Check sheet for the drawn part. Datum: minimum x, y, z corner. Units: mm. A direction names the side the tool comes from. Coordinates: 2 decimals unless noted, no trailing zeros. Order: outer loops, then holes, each group sorted by start corner. A loop starts at its lowest first (then second) coordinate and runs counter-clockwise, first axis right, second up. Notation, with made-up numbers: (65, -12.75) -> (110, -12.75) arc R20 ccw to (110, 2.25) -> close; hole circle Ø11 at (-11.5, 5.5). An arc over 180 degrees is marked (long way). Write item = value, one per line. Start each with the question number.
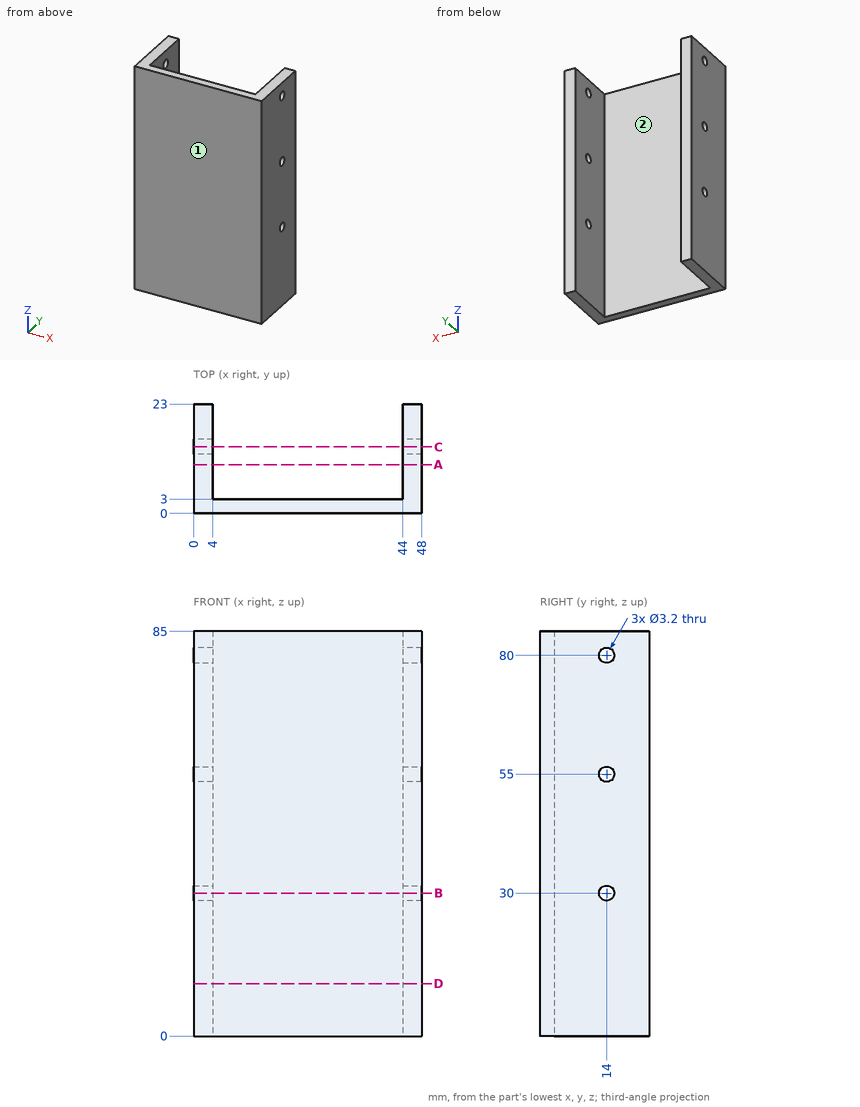
Item 1: Thickness scan on line 1 (Y direction, x = 2.7, z = 55); line 2 (X direction, y = 7, z = 33); line 3 (Y direction, x = 22.5, z = 27). Record the ranges inside material, lowest first.
Item 2: Section check C-C (y = 14). State how many separate pieces and enclosed holes the cut face has, then the cut area to 3 significant figures.
Item 3: Tool access check on the marked faces 1 and 2. Record the directions out of +Z, -Z, +X, -X, +Y, -Y that give a thin tool (end or side, any length) a straight path to the whole face; none if there is none.
Item 4: Section check B-B (z = 30). Record the boundary of the cut face in (x, y).
Item 5: Section check A-A (y = 10.25). Record the boundary of the cut face in (x, z), then the cut area to 3 significant figures.
Item 6: Gauge pin test, flat ends, axial feed: P1, Ø10, axis at x = 21, z = 9.5, coming from the +Y side; P2, Ø1, axis at x = 5.5, y = 18, coming from the +Z side. Record the tip position at first contact, or that the pin passes through.
Item 7: Section check D-D (z = 11). Record the boundary of the cut face in (x, y), then the cut area to 3 significant figures.
Filled sheet:
q1.line_1 = 0 to 12.4, 15.6 to 23
q1.line_2 = 0 to 4, 44 to 48
q1.line_3 = 0 to 3
q2.separate_pieces = 8
q2.enclosed_holes = 0
q2.area = 603 mm^2
q3.face_1 = +Z, -Z, +X, -X, -Y
q3.face_2 = +Z, -Z, +Y
q4.outline = (0, 0) -> (48, 0) -> (48, 12.4) -> (44, 12.4) -> (44, 3) -> (4, 3) -> (4, 12.4) -> (0, 12.4) -> close; (0, 15.6) -> (4, 15.6) -> (4, 23) -> (0, 23) -> close; (44, 15.6) -> (48, 15.6) -> (48, 23) -> (44, 23) -> close
q5.outline = (0, 0) -> (4, 0) -> (4, 85) -> (0, 85) -> close; (44, 0) -> (48, 0) -> (48, 85) -> (44, 85) -> close
q5.area = 680 mm^2
q6.P1 = 3
q6.P2 = through
q7.outline = (0, 0) -> (48, 0) -> (48, 23) -> (44, 23) -> (44, 3) -> (4, 3) -> (4, 23) -> (0, 23) -> close
q7.area = 304 mm^2
